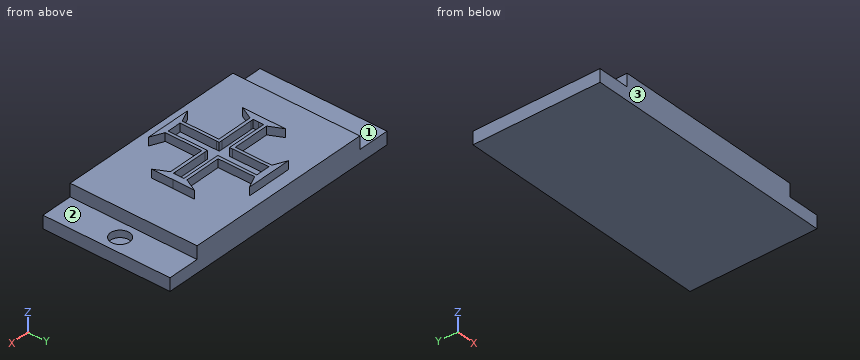
```python
from build123d import *

# Parameters (mm, degrees)
F0_W     = 30
F0_H     = 20
F1_DEPTH = 4
F2_W     = 5
F2_H     = 20
F3_DEPTH = 2
F5_DEPTH = 1.3
F6_W     = 5
F6_H     = 20
F7_DEPTH = 2
F8_R     = 1.5
F9_DEPTH = 1.1


with BuildPart() as f1:
    # F0 (on Top) → F1 (new body)
    with BuildSketch(Plane.XY):
        with Locations((-15, 10)):
            Rectangle(F0_W, F0_H)
    extrude(amount=F1_DEPTH)

    # F2 (on face) → F3 (join)
    with BuildSketch(Plane(origin=(0, 0, 0), x_dir=(1, 0, 0), z_dir=(0, 0, -1))):
        with Locations((-32.5, -10)):
            Rectangle(F2_W, F2_H)
    extrude(amount=-F3_DEPTH)

    # F4 (on face) → F5 (join)
    with BuildSketch(Plane.XY.offset(4)):
        Polygon((-14.4567919296, 10.897058451), (-13.9734713034, 10.8974938178), (-13.9741291965, 11.3685017389), (-14.4561063498, 11.3666541874), align=None)
        Polygon((-13.9741291965, 11.3685017389), (-13.9734713034, 10.8974938178), (-8.5701756179, 10.902361013), (-8.198968805, 10.9070869228), (-8.1985752936, 10.0812381133), (-8.198968805, 9.2553893039), (-8.5701756179, 9.2601152137), (-13.9734713034, 9.2649824089), (-13.9741291965, 8.7939744878), (-8.2043278962, 8.7718572468), (-7.1527287364, 6.6936984658), (-7.1703906207, 10.0812381133), (-7.1527287364, 13.4687777609), (-8.2043278962, 11.3906189799), align=None)
        Polygon((-14.4561063498, 11.3666541874), (-13.9741291965, 11.3685017389), (-13.9821750256, 17.1287826718), (-11.9453166755, 18.0399830909), (-15.5499000102, 18.0399830909), (-19.1544833449, 18.0399830909), (-17.1176249949, 17.1287826718), (-17.1256708239, 11.3685017389), (-16.6436936706, 11.3666541874), (-16.6520233348, 17.0721532121), (-16.650039608, 17.0703820259), (-15.5499000102, 17.0703820259), (-14.4497604124, 17.0703820259), (-14.4477766856, 17.0721532121), align=None)
        Polygon((-13.9741291965, 8.7939744878), (-13.9734713034, 9.2649824089), (-14.4567919296, 9.2654177757), (-14.4561063498, 8.7958220392), align=None)
        Polygon((-16.6436936706, 11.3666541874), (-17.1256708239, 11.3685017389), (-17.1263287171, 10.8974938178), (-16.6430080908, 10.897058451), align=None)
        Polygon((-17.1263287171, 10.8974938178), (-17.1256708239, 11.3685017389), (-22.8954721242, 11.3906189799), (-23.9470712841, 13.4687777609), (-23.9294093997, 10.0812381133), (-23.9470712841, 6.6936984658), (-22.8954721242, 8.7718572468), (-17.1256708239, 8.7939744878), (-17.1263287171, 9.2649824089), (-22.5296244025, 9.2601152137), (-22.9008312154, 9.2553893039), (-22.9012247269, 10.0812381133), (-22.9008312154, 10.9070869228), (-22.5296244025, 10.902361013), align=None)
        Polygon((-13.9821750256, 3.0336935549), (-13.9741291965, 8.7939744878), (-14.4561063498, 8.7958220392), (-14.4477766856, 3.0903230146), (-14.4497604124, 3.0920942008), (-15.5499000102, 3.0920942008), (-16.650039608, 3.0920942008), (-16.6520233348, 3.0903230146), (-16.6436936706, 8.7958220392), (-17.1256708239, 8.7939744878), (-17.1176249949, 3.0336935549), (-19.1544833449, 2.1224931358), (-15.5499000102, 2.1224931358), (-11.9453166755, 2.1224931358), align=None)
        Polygon((-17.1263287171, 9.2649824089), (-17.1256708239, 8.7939744878), (-16.6436936706, 8.7958220392), (-16.6430080908, 9.2654177757), align=None)
    extrude(amount=F5_DEPTH)

    # F6 (on face) → F7 (join)
    with BuildSketch(Plane(origin=(0, 0, 0), x_dir=(1, 0, 0), z_dir=(0, 0, -1))):
        with Locations((2.5, -10)):
            Rectangle(F6_W, F6_H)
    extrude(amount=-F7_DEPTH)

    # F8 (on face) → F9 (cut)
    with BuildSketch(Plane.XY.offset(2)):
        with Locations((2.5, 10)):
            Circle(F8_R)
    extrude(amount=-F9_DEPTH, mode=Mode.SUBTRACT)


solid = f1.part
```
Model file for the job. Use its own axes, mm. Face numbers are marked on the shaded views. A direction names the side the tool comes from. Coordinates: 2 decimals unless noted, no trailing zeros. Order: outer loops, then holes, each group sorted by start corner. A loop starts at its lowest first (then second) coordinate and runs counter-clockwise, first axis right, second up. Notation, with made-up numbers: (-26.75, 66) - (-19.75, 66) arc R16 cw to (-19.75, 96) - close; hole circle Ø8 at (11.25, 42). An arc over 180 degrees is marked (long way). Return JSON: item names as keys, results as strings. Group by question number.
1) Tool access for the marked faces 1, 2 and 3: list every direction of +Z, -Z, +X, -X, +Y, -Y with a clear straight run to the whole face (end or side of a thin tool).
2) Saw through at D-D, the plane x = -13. Write the cut outline in (y, z), plus the area to 3 significant figures.
3) Flat gauge pins, fed straight in: P1, Ø0.6, axis at x = -16, z = 4.5, coming from the +Y side; P2, Ø2.5, axis at x = 2.5, y = 8.5, coming from the +Z side; P3, Ø1.5, axis at y = 16.5, z = 3.5, coming from the +X side. Where does each tip first touch, or does it go through?
4) Saw through at B-B, the plane y = 18.5. Write the cut outline in (x, z), plus the area to 3 significant figures.
5) Saw through at A-A, the plane x = 2.5. Write the cut outline in (y, z), plus the area to 3 significant figures.
6) Probe line 1 (Y direction, x = 2.5, z = 1.1); line 2 (X direction, y = 15.5, z = 4.9). List the from-to ranges inside material, lowest first. Write a range as from..to.
7) Saw through at C-C, the plane z = 2.4. Write the cut outline in (x, y).
Values found:
{
 "1": {"face 1": "+Z, -X, +Y, -Y", "face 2": "+Z, +X, +Y, -Y", "face 3": "+Z, -Z, +X, -X, -Y"},
 "2": {"outline": "(0, 0) - (20, 0) - (20, 4) - (18.04, 4) - (18.04, 5.3) - (17.57, 5.3) - (17.57, 4) - (11.37, 4) - (11.37, 5.3) - (10.9, 5.3) - (10.9, 4) - (9.26, 4) - (9.26, 5.3) - (8.79, 5.3) - (8.79, 4) - (2.59, 4) - (2.59, 5.3) - (2.12, 5.3) - (2.12, 4) - (0, 4) - close", "area": "82.5 mm²"},
 "3": {"P1": "stops at y = 18.04", "P2": "stops at z = 2", "P3": "stops at x = 0"},
 "4": {"outline": "(-35, 0) - (5, 0) - (5, 2) - (0, 2) - (0, 4) - (-30, 4) - (-30, 2) - (-35, 2) - close", "area": "140 mm²"},
 "5": {"outline": "(0, 0) - (20, 0) - (20, 2) - (11.5, 2) - (11.5, 0.9) - (8.5, 0.9) - (8.5, 2) - (0, 2) - close", "area": "36.7 mm²"},
 "6": {"line 1": "y = 0..8.5, 11.5..20", "line 2": "x = -17.12..-16.65, -14.45..-13.98"},
 "7": {"outline": "(-30, 0) - (0, 0) - (0, 20) - (-30, 20) - close"}
}
